Read the model definition and answer for the solid it produces. Units are mm, in the model's axes. A direction names the side the tool comes from. Coordinates: 2 decimals unless noted, no trailing zeros. Write each loop counter-clockwise with the first axis right and the second up, starting at its lowest first coordinate (ties: lowest second). Pieces come first, ordered by that corner, then holes.
1) Determine the mould class of faces 1 (the face through (9, -25, 0)), 2 (the face through (10.9, -37.6, -8)), 3 (the face through (8.642, -4.056, -37.273)) for opening direction Z: +Z half, -Z half, draft (parallel to the pull), parting line (faces both ways), or undercut.
2) Find the intervals of material crossed by line 1 (Y direction, x = 9, z = -3.5); line 2 (Z direction, x = 3.25, y = -31.5), in increasing order.
3) Which of the six approach directions +Z, -Z, +X, -X, +Y, -Y give full straight-line access (tool end or side, diameter ignored) to faces 4 (the face through (10.9, -8, -42.4)), 5 (the face through (0, -20, -14))?
4) This flat-tipped pin is pushed along its axis until it touches: pin 1 Ø5 at (x, y) = (4.5, -33.5) entering from -Z. Where does it stop, or does it pass through?
5) The part is cut by section B-B (z = -40). Determine the outline of the cut face in (x, y), then the cut area to 3 significant figures.
6) The part is cut by section D-D (x = 16). Determine the outline of the cut face in (y, z), then the cut area to 3 significant figures.
7) The part is cut by section A-A (x = 9). Determine the outline of the cut face in (y, z).
Autodesk Inventor part; units mm, degrees
ref_plane "YZ Plane" through (0, 0, 0) normal (1, 0, 0) x (0, 1, 0)
ref_plane "XZ Plane" through (0, 0, 0) normal (0, 1, 0) x (-1, 0, 0)
ref_plane "XY Plane" through (0, 0, 0) normal (0, 0, 1) x (1, 0, 0)
sketch "Sketch1" plane through (0, 0, 0) normal (1, 0, 0) x (0, 1, 0)
  line L0 (-50, 0) -> (0, 0)
  line L1 (0, 0) -> (0, -50)
  line L2 (0, -50) -> (-8, -50)
  line L3 (-8, -50) -> (-8, -30)
  line L4 (-8, -30) -> (-30, -8)
  line L5 (-30, -8) -> (-50, -8)
  line L6 (-50, -8) -> (-50, 0)
  dimension "d0" = 50
  dimension "d1" = 8
  dimension "d2" = 8
  dimension "d3" = 20
  dimension "d4" = 20
extrude "Extrusion1" add sketch "Sketch1" along normal blind 18
sketch "Sketch2" plane through (0, -8, -50) normal (0, -1, 0) x (1, 0, 0)
  circle A0 centre (9, 10) radius 2.75
  line L0 (18, 20) -> (18, 0)
  line L1 (0, 0) -> (18, 0)
  point P0 (0, 50)
  dimension "d7" = 5.5
  dimension "d8" = 9
  dimension "d9" = 10
extrude "Extrusion2" cut sketch "Sketch2" against normal through all
sketch "Sketch3" plane through (0, -50, -8) normal (0, 0, -1) x (-1, 0, 0)
  circle A0 centre (-9, 10) radius 2.75
  line L0 (-18, 0) -> (-18, 20)
  line L1 (0, 0) -> (-18, 0)
  point P0 (0, 50)
  dimension "d12" = 5.5
  dimension "d13" = 9
  dimension "d14" = 10
extrude "Extrusion3" cut sketch "Sketch3" against normal through all
properties part number "90degree Braces" material "Steel, Cast"
Reported:
1. face 1: +Z half
1. face 2: -Z half
1. face 3: undercut
2. line 1: y = -50 to -42.75, -37.25 to 0
2. line 2: z = -8 to 0
3. face 4: -Z, +X, -X, -Y
3. face 5: +Z, -Z, -X, +Y, -Y
4. pin 1: stops at z = -8
5. outline: (0, -8) - (6.25, -8) - (6.25, 0) - (0, 0) - close; (11.75, -8) - (18, -8) - (18, 0) - (11.75, 0) - close
5. area: 100 mm2
6. outline: (-50, -8) - (-30, -8) - (-8, -30) - (-8, -50) - (0, -50) - (0, 0) - (-50, 0) - close
6. area: 978 mm2
7. outline: (-50, -8) - (-42.75, -8) - (-42.75, 0) - (-50, 0) - close; (-37.25, -8) - (-30, -8) - (-8, -30) - (-8, -37.25) - (0, -37.25) - (0, 0) - (-37.25, 0) - close; (-8, -50) - (0, -50) - (0, -42.75) - (-8, -42.75) - close
